Work out the finished part from the listing and answer in its coordinate system (mm). Face numbers are marked on the shaded views. Round coordinates to 2 decimals unless told otherwise and drop trailing zeros. Order: outer loops, then holes, each group sorted by start corner. A loop starts at its lowest first (then second) coordinate and runs counter-clockwise, first axis right, second up. Notation, with made-up numbers: M 54.25,59.25 L 66.25,59.25 A37 cw 66.25,97.25 Z; hole C 26,48 d4. An arc over 180 degrees is marked long. Return JSON: item names as keys, results as strings.
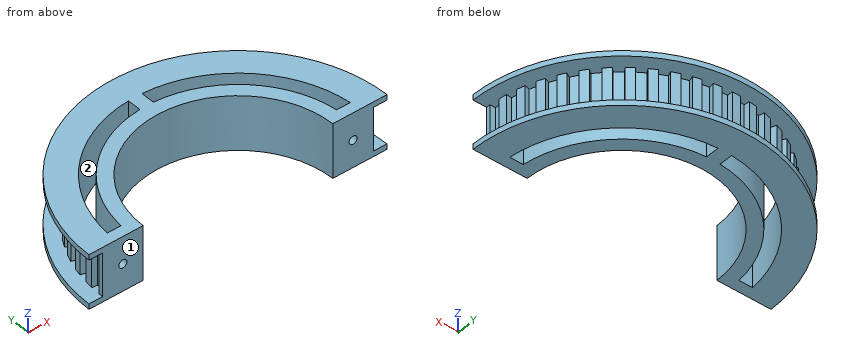
from build123d import *

# Parameters (mm, degrees)
BOSS_EXTRUDE1_DEPTH = 20
CUT_EXTRUDE2_REACH  = 75.453
SKETCH3_R           = 1.5
BOSS_EXTRUDE3_DEPTH = 2
BOSS_EXTRUDE4_START = -2
BOSS_EXTRUDE4_DEPTH = 2


with BuildPart() as part:
    # Sketch1 → Boss-Extrude1 (new body)
    with BuildSketch(Plane.XY):
        with BuildLine():
            Line((35, 0), (49.976556775, 0))
            Line((49.976556775, 0), (49.976556775, 1.5))
            Line((49.976556775, 1.5), (47.976556775, 1.5))
            ThreePointArc((47.976556775, 1.5), (47.897228315, 3.139350203), (47.761899969, 4.77502998))
            Line((47.761899969, 4.77502998), (49.744789692, 5.036082364))
            Line((49.744789692, 5.036082364), (49.353211116, 8.010416948))
            Line((49.353211116, 8.010416948), (47.370321393, 7.749364564))
            ThreePointArc((47.370321393, 7.749364564), (47.077693459, 9.364335457), (46.730023813, 10.968357872))
            Line((46.730023813, 10.968357872), (48.661875466, 11.485995963))
            Line((48.661875466, 11.485995963), (47.88541833, 14.383773441))
            Line((47.88541833, 14.383773441), (45.953566678, 13.866135351))
            ThreePointArc((45.953566678, 13.866135351), (45.452646216, 15.429094335), (44.898583993, 16.974014121))
            Line((44.898583993, 16.974014121), (46.746343059, 17.739380986))
            Line((46.746343059, 17.739380986), (45.598292761, 20.511019583))
            Line((45.598292761, 20.511019583), (43.750533696, 19.745652719))
            ThreePointArc((43.750533696, 19.745652719), (43.049891594, 21.229857131), (42.298916953, 22.689240282))
            Line((42.298916953, 22.689240282), (44.030967761, 23.689240282))
            Line((44.030967761, 23.689240282), (42.530967761, 26.287316493))
            Line((42.530967761, 26.287316493), (40.798916953, 25.287316493))
            ThreePointArc((40.798916953, 25.287316493), (39.910541391, 26.667371185), (38.975503717, 28.016247251))
            Line((38.975503717, 28.016247251), (40.562210397, 29.233770109))
            Line((40.562210397, 29.233770109), (38.73592611, 31.61383013))
            Line((38.73592611, 31.61383013), (37.14921943, 30.396307272))
            ThreePointArc((37.14921943, 30.396307272), (36.088310759, 31.648599125), (34.985208805, 32.863888462))
            Line((34.985208805, 32.863888462), (36.399422368, 34.278102024))
            Line((36.399422368, 34.278102024), (34.278102024, 36.399422368))
            Line((34.278102024, 36.399422368), (32.863888462, 34.985208805))
            ThreePointArc((32.863888462, 34.985208805), (31.648599125, 36.088310759), (30.396307272, 37.14921943))
            Line((30.396307272, 37.14921943), (31.61383013, 38.73592611))
            Line((31.61383013, 38.73592611), (29.233770109, 40.562210397))
            Line((29.233770109, 40.562210397), (28.016247251, 38.975503717))
            ThreePointArc((28.016247251, 38.975503717), (26.667371185, 39.910541391), (25.287316493, 40.798916953))
            Line((25.287316493, 40.798916953), (26.287316493, 42.530967761))
            Line((26.287316493, 42.530967761), (23.689240282, 44.030967761))
            Line((23.689240282, 44.030967761), (22.689240282, 42.298916953))
            ThreePointArc((22.689240282, 42.298916953), (21.229857131, 43.049891594), (19.745652719, 43.750533696))
            Line((19.745652719, 43.750533696), (20.511019583, 45.598292761))
            Line((20.511019583, 45.598292761), (17.739380986, 46.746343059))
            Line((17.739380986, 46.746343059), (16.974014121, 44.898583993))
            ThreePointArc((16.974014121, 44.898583993), (15.429094335, 45.452646216), (13.866135351, 45.953566678))
            Line((13.866135351, 45.953566678), (14.383773441, 47.88541833))
            Line((14.383773441, 47.88541833), (11.485995963, 48.661875466))
            Line((11.485995963, 48.661875466), (10.968357872, 46.730023813))
            ThreePointArc((10.968357872, 46.730023813), (9.364335457, 47.077693459), (7.749364564, 47.370321393))
            Line((7.749364564, 47.370321393), (8.010416948, 49.353211116))
            Line((8.010416948, 49.353211116), (5.036082364, 49.744789692))
            Line((5.036082364, 49.744789692), (4.77502998, 47.761899969))
            ThreePointArc((4.77502998, 47.761899969), (3.139350203, 47.897228315), (1.5, 47.976556775))
            Line((1.5, 47.976556775), (1.5, 49.976556775))
            Line((1.5, 49.976556775), (-1.5, 49.976556775))
            Line((-1.5, 49.976556775), (-1.5, 47.976556775))
            ThreePointArc((-1.5, 47.976556775), (-3.139350203, 47.897228315), (-4.77502998, 47.761899969))
            Line((-4.77502998, 47.761899969), (-5.036082364, 49.744789692))
            Line((-5.036082364, 49.744789692), (-8.010416948, 49.353211116))
            Line((-8.010416948, 49.353211116), (-7.749364564, 47.370321393))
            ThreePointArc((-7.749364564, 47.370321393), (-9.364335457, 47.077693459), (-10.968357872, 46.730023813))
            Line((-10.968357872, 46.730023813), (-11.485995963, 48.661875466))
            Line((-11.485995963, 48.661875466), (-14.383773441, 47.88541833))
            Line((-14.383773441, 47.88541833), (-13.866135351, 45.953566678))
            ThreePointArc((-13.866135351, 45.953566678), (-15.429094335, 45.452646216), (-16.974014121, 44.898583993))
            Line((-16.974014121, 44.898583993), (-17.739380986, 46.746343059))
            Line((-17.739380986, 46.746343059), (-20.511019583, 45.598292761))
            Line((-20.511019583, 45.598292761), (-19.745652719, 43.750533696))
            ThreePointArc((-19.745652719, 43.750533696), (-21.229857131, 43.049891594), (-22.689240282, 42.298916953))
            Line((-22.689240282, 42.298916953), (-23.689240282, 44.030967761))
            Line((-23.689240282, 44.030967761), (-26.287316493, 42.530967761))
            Line((-26.287316493, 42.530967761), (-25.287316493, 40.798916953))
            ThreePointArc((-25.287316493, 40.798916953), (-26.667371185, 39.910541391), (-28.016247251, 38.975503717))
            Line((-28.016247251, 38.975503717), (-29.233770109, 40.562210397))
            Line((-29.233770109, 40.562210397), (-31.61383013, 38.73592611))
            Line((-31.61383013, 38.73592611), (-30.396307272, 37.14921943))
            ThreePointArc((-30.396307272, 37.14921943), (-31.648599125, 36.088310759), (-32.863888462, 34.985208805))
            Line((-32.863888462, 34.985208805), (-34.278102024, 36.399422368))
            Line((-34.278102024, 36.399422368), (-36.399422368, 34.278102024))
            Line((-36.399422368, 34.278102024), (-34.985208805, 32.863888462))
            ThreePointArc((-34.985208805, 32.863888462), (-36.088310759, 31.648599125), (-37.14921943, 30.396307272))
            Line((-37.14921943, 30.396307272), (-38.73592611, 31.61383013))
            Line((-38.73592611, 31.61383013), (-40.562210397, 29.233770109))
            Line((-40.562210397, 29.233770109), (-38.975503717, 28.016247251))
            ThreePointArc((-38.975503717, 28.016247251), (-39.910541391, 26.667371185), (-40.798916953, 25.287316493))
            Line((-40.798916953, 25.287316493), (-42.530967761, 26.287316493))
            Line((-42.530967761, 26.287316493), (-44.030967761, 23.689240282))
            Line((-44.030967761, 23.689240282), (-42.298916953, 22.689240282))
            ThreePointArc((-42.298916953, 22.689240282), (-43.049891594, 21.229857131), (-43.750533696, 19.745652719))
            Line((-43.750533696, 19.745652719), (-45.598292761, 20.511019583))
            Line((-45.598292761, 20.511019583), (-46.746343059, 17.739380986))
            Line((-46.746343059, 17.739380986), (-44.898583993, 16.974014121))
            ThreePointArc((-44.898583993, 16.974014121), (-45.452646216, 15.429094335), (-45.953566678, 13.866135351))
            Line((-45.953566678, 13.866135351), (-47.88541833, 14.383773441))
            Line((-47.88541833, 14.383773441), (-48.661875466, 11.485995963))
            Line((-48.661875466, 11.485995963), (-46.730023813, 10.968357872))
            ThreePointArc((-46.730023813, 10.968357872), (-47.077693459, 9.364335457), (-47.370321393, 7.749364564))
            Line((-47.370321393, 7.749364564), (-49.353211116, 8.010416948))
            Line((-49.353211116, 8.010416948), (-49.744789692, 5.036082364))
            Line((-49.744789692, 5.036082364), (-47.761899969, 4.77502998))
            ThreePointArc((-47.761899969, 4.77502998), (-47.897228315, 3.139350203), (-47.976556775, 1.5))
            Line((-47.976556775, 1.5), (-49.976556775, 1.5))
            Line((-49.976556775, 1.5), (-49.976556775, 0))
            Line((-49.976556775, 0), (-35, 0))
            ThreePointArc((-35, 0), (0, 35), (35, 0))
        make_face()
        with BuildLine():
            Line((44.821869662, 4), (39.799497484, 4))
            ThreePointArc((39.799497484, 4), (27.747175978, 28.811355839), (2.5, 39.921798557))
            Line((2.5, 39.921798557), (2.5, 44.930501889))
            ThreePointArc((2.5, 44.930501889), (31.283643223, 32.34708127), (44.821869662, 4))
        make_face(mode=Mode.SUBTRACT)
        with BuildLine():
            ThreePointArc((-44.821869662, 4), (-31.283643223, 32.34708127), (-2.5, 44.930501889))
            Line((-2.5, 44.930501889), (-2.5, 39.921798557))
            ThreePointArc((-2.5, 39.921798557), (-27.747175978, 28.811355839), (-39.799497484, 4))
            Line((-39.799497484, 4), (-44.821869662, 4))
        make_face(mode=Mode.SUBTRACT)
    extrude(amount=BOSS_EXTRUDE1_DEPTH)

    # Sketch3 → Cut-Extrude2 (cut, up to next)
    with BuildSketch(Plane.XZ, mode=Mode.PRIVATE) as cut_extrude2_sk1:
        with Locations(Location((-42.5, 10, 0), (0, 0, 270))):
            Circle(SKETCH3_R)
    cut_extrude2_tool1 = extrude(cut_extrude2_sk1.sketch, amount=-CUT_EXTRUDE2_REACH, mode=Mode.PRIVATE) & part.part
    cut_extrude2 = cut_extrude2_tool1.solids().sort_by_distance((-42.5, 0, 10))[0]
    add(cut_extrude2, mode=Mode.SUBTRACT)

    # Mirror2: Cut-Extrude2 across plane
    add(cut_extrude2.mirror(Plane(origin=(0, 0, 0), x_dir=(0, 0, 1), z_dir=(1, 0, 0))), mode=Mode.SUBTRACT)

    # Sketch5 → Boss-Extrude3 (add)
    with BuildSketch(Plane.XY):
        with BuildLine():
            Line((-48, 0), (-55, 0))
            ThreePointArc((-55, 0), (0, 55), (55, 0))
            Line((55, 0), (48, 0))
            ThreePointArc((48, 0), (0, 48), (-48, 0))
        make_face()
    extrude(amount=BOSS_EXTRUDE3_DEPTH)

    # Sketch6 → Boss-Extrude4 (add)
    with BuildSketch(Plane.XY.offset(20).offset(BOSS_EXTRUDE4_START)):
        with BuildLine():
            Line((-45, 0), (-55, 0))
            ThreePointArc((-55, 0), (0, 55), (55, 0))
            Line((55, 0), (45, 0))
            ThreePointArc((45, 0), (0, 45), (-45, 0))
        make_face()
    extrude(amount=BOSS_EXTRUDE4_DEPTH)


solid = part.part
Item 1: The mould has two halves that part along X. Classify the marked faces 1 and 2: pulls with the +X half, pulls with the -X half, needs draft (parallel to the pull), parting line crosses it, or undercut.
Output:
{"face 1": "needs draft", "face 2": "undercut"}
Item 2: Find section A-A (x = 0). Determine the outline of the cut face in (y, z).
Output:
{"outline": "M 35,0 L 55,0 L 55,2 L 49.98,2 L 49.98,18 L 55,18 L 55,20 L 35,20 Z"}
Item 3: Each of these flat-tipped pins is pushed along its axis until it touches: pin 1 (1.5 mm diameter, centred on y = 43, z = 11.5, fed in from -X); pin 2 (1 mm diameter, centred on x = -5.5, z = 14.5, fed in from +Y); pin 3 (4 mm diameter, centred on y = 24, z = 10.5, fed in from +X). Where does it stop, or does it pass through?
Output:
{"pin 1": "stops at x = -26.29", "pin 2": "stops at y = 49.74", "pin 3": "stops at x = 44.03"}
Item 4: Find section B-B (z = 3.25). State how many separate pieces and enclosed holes the cut face has, plus the area to 3 significant figures.
Output:
{"separate pieces": "1", "enclosed holes": "2", "area": "1,240 mm^2"}
Item 5: Consider line 1 along X through (y, z) = (0.8, 10); line 2 along Z through (x, y) = (-18, 51); line 3 along X through (y, z) = (15, 7.75). Determine where each line is inside the solid, lowest interval first. Write a range as [from, to].
Output:
{"line 1": "x = [-49.98, -44], [-41, -34.99], [34.99, 41], [44, 49.98]", "line 2": "z = [0, 2], [18, 20]", "line 3": "x = [-45.6, -42.43], [-37.08, -31.62], [31.62, 37.08], [42.43, 45.6]"}
